Check sheet for the modelled part. Datum: model origin and axes. Units: mm. A direction names the side the tool comes from. Give positions to 0.01 mm unless a question says otherwise; leave off trailing zeros. Write each question's results on one line, items separated by ' | '. Start each with the question number.
1. Tool access check on faces 1 (the face through (88, 34, -49)), 2 (the face through (90, 26, -49)), 3 (the face through (52, 45.7, -49)). Record the directions out of +Z, -Z, +X, -X, +Y, -Y that give a thin tool (end or side, any length) a straight path to the whole face; none if there is none.
2. Material ranges on L1, parallel to Y at x = 77.5, z = -93.5; L2, parallel to Y at x = 47, z = -74.5; L3, parallel to Y at x = 59, z = -47.5, recorded low to high. Write a range as from..to.
3. Gauge pin test, flat ends, axial feed: pin 1 Ø6 at (x, y) = (82, 16) entering from -Z; pin 2 Ø10 at (x, z) = (56, -46.5) entering from +Y; pin 3 Ø2 at (y, z) = (3, -56) entering from -X; pin 4 Ø1.6 at (x, z) = (58.5, -64) entering from +Y. Record the tip position at first contact, or that the pin passes through.
4. Mould release check, pull along Y, two halves, no side actions. Record for faces 4 (the face through (52.82, 48, -49)), 5 (the face through (80, 1.83, -49)), 6 (the face through (87, 50.35, -49)): +Y half, -Y half, draft (parallel to the pull), parting line (faces both ways), or undercut.
from build123d import *

# Parameters (mm, degrees)
BOSS_EXTRUDE1_DEPTH = 100


with BuildPart() as part:
    # Sketch2 → Boss-Extrude1 (new body)
    with BuildSketch(Plane(origin=(0, 0, 0), x_dir=(-1, 0, 0), z_dir=(0, 0, -1))):
        with BuildLine():
            Line((-81.1, 43.92), (-46.615, 43.92))
            Line((-46.615, 43.92), (-46.615, 45.7))
            Line((-46.615, 45.7), (-49, 45.7))
            Line((-49, 45.7), (-49, 48.57))
            Line((-49, 48.57), (-45, 48.57))
            Line((-45, 48.57), (-45, 50.35))
            Line((-45, 50.35), (-50.82, 50.35))
            Line((-50.82, 50.35), (-50.82, 45.7))
            Line((-50.82, 45.7), (-52.82, 45.7))
            Line((-52.82, 45.7), (-52.82, 50.35))
            Line((-52.82, 50.35), (-54.224444444, 50.35))
            Line((-54.224444444, 50.35), (-54.224444444, 45.7))
            Line((-54.224444444, 45.7), (-56.224444444, 45.7))
            Line((-56.224444444, 45.7), (-56.224444444, 50.35))
            Line((-56.224444444, 50.35), (-57.628888889, 50.35))
            Line((-57.628888889, 50.35), (-57.628888889, 45.7))
            Line((-57.628888889, 45.7), (-59.628888889, 45.7))
            Line((-59.628888889, 45.7), (-59.628888889, 50.35))
            Line((-59.628888889, 50.35), (-61.033333333, 50.35))
            Line((-61.033333333, 50.35), (-61.033333333, 45.7))
            Line((-61.033333333, 45.7), (-63.033333333, 45.7))
            Line((-63.033333333, 45.7), (-63.033333333, 50.35))
            Line((-63.033333333, 50.35), (-64.437777778, 50.35))
            Line((-64.437777778, 50.35), (-64.437777778, 45.7))
            Line((-64.437777778, 45.7), (-66.437777778, 45.7))
            Line((-66.437777778, 45.7), (-66.437777778, 50.35))
            Line((-66.437777778, 50.35), (-67.842222222, 50.35))
            Line((-67.842222222, 50.35), (-67.842222222, 45.7))
            Line((-67.842222222, 45.7), (-69.842222222, 45.7))
            Line((-69.842222222, 45.7), (-69.842222222, 50.35))
            Line((-69.842222222, 50.35), (-71.246666667, 50.35))
            Line((-71.246666667, 50.35), (-71.246666667, 45.7))
            Line((-71.246666667, 45.7), (-73.246666667, 45.7))
            Line((-73.246666667, 45.7), (-73.246666667, 50.35))
            Line((-73.246666667, 50.35), (-74.651111111, 50.35))
            Line((-74.651111111, 50.35), (-74.651111111, 45.7))
            Line((-74.651111111, 45.7), (-76.651111111, 45.7))
            Line((-76.651111111, 45.7), (-76.651111111, 50.35))
            Line((-76.651111111, 50.35), (-78.055555556, 50.35))
            Line((-78.055555556, 50.35), (-78.055555556, 45.7))
            Line((-78.055555556, 45.7), (-80.055555556, 45.7))
            Line((-80.055555556, 45.7), (-80.055555556, 50.35))
            Line((-80.055555556, 50.35), (-81.46, 50.35))
            Line((-81.46, 50.35), (-81.46, 46.490680448))
            Line((-81.46, 46.490680448), (-83.46, 47.61664944))
            Line((-83.46, 47.61664944), (-83.46, 50.35))
            Line((-83.46, 50.35), (-90, 50.35))
            Line((-90, 50.35), (-90, 0))
            Line((-90, 0), (-72.9, 0))
            Line((-72.9, 0), (-72.9, 1.83))
            Line((-72.9, 1.83), (-74.3, 1.83))
            Line((-74.3, 1.83), (-74.3, 4.2))
            Line((-74.3, 4.2), (-67.3, 4.2))
            Line((-67.3, 4.2), (-67.3, 1.83))
            Line((-67.3, 1.83), (-68.7, 1.83))
            Line((-68.7, 1.83), (-68.7, 0))
            Line((-68.7, 0), (-45, 0))
            Line((-45, 0), (-45, 1.83))
            Line((-45, 1.83), (-65.3, 1.83))
            Line((-65.3, 1.83), (-65.3, 6.2))
            Line((-65.3, 6.2), (-77.73, 6.2))
            Line((-77.73, 6.2), (-77.73, 4.2))
            Line((-77.73, 4.2), (-76.3, 4.2))
            Line((-76.3, 4.2), (-76.3, 1.83))
            Line((-76.3, 1.83), (-83.3, 1.83))
            Line((-83.3, 1.83), (-83.3, 4.2))
            Line((-83.3, 4.2), (-81.87, 4.2))
            Line((-81.87, 4.2), (-81.87, 6.2))
            Line((-81.87, 6.2), (-84.76556902, 6.2))
            Line((-84.76556902, 6.2), (-85.557358859, 4.697239063))
            ThreePointArc((-85.557358859, 4.697239063), (-86.149971444, 2.200236409), (-86.836478439, 4.673072852))
            Line((-86.836478439, 4.673072852), (-88, 6.6925))
            Line((-88, 6.6925), (-86.26, 6.6925))
            Line((-86.26, 6.6925), (-86.26, 8.23))
            Line((-86.26, 8.23), (-88, 8.23))
            Line((-88, 8.23), (-88, 10.19))
            Line((-88, 10.19), (-86.26, 10.19))
            Line((-86.26, 10.19), (-86.26, 11.7275))
            Line((-86.26, 11.7275), (-88, 11.7275))
            Line((-88, 11.7275), (-88, 13.6875))
            Line((-88, 13.6875), (-86.26, 13.6875))
            Line((-86.26, 13.6875), (-86.26, 15.225))
            Line((-86.26, 15.225), (-88, 15.225))
            Line((-88, 15.225), (-88, 17.185))
            Line((-88, 17.185), (-86.26, 17.185))
            Line((-86.26, 17.185), (-86.26, 18.7225))
            Line((-86.26, 18.7225), (-88, 18.7225))
            Line((-88, 18.7225), (-88, 20.6825))
            Line((-88, 20.6825), (-86.26, 20.6825))
            Line((-86.26, 20.6825), (-86.26, 22.22))
            Line((-86.26, 22.22), (-88, 22.22))
            Line((-88, 22.22), (-88, 24.18))
            Line((-88, 24.18), (-86.26, 24.18))
            Line((-86.26, 24.18), (-86.26, 25.7175))
            Line((-86.26, 25.7175), (-88, 25.7175))
            Line((-88, 25.7175), (-88, 27.6775))
            Line((-88, 27.6775), (-86.26, 27.6775))
            Line((-86.26, 27.6775), (-86.26, 29.215))
            Line((-86.26, 29.215), (-88, 29.215))
            Line((-88, 29.215), (-88, 31.175))
            Line((-88, 31.175), (-86.26, 31.175))
            Line((-86.26, 31.175), (-86.26, 32.7125))
            Line((-86.26, 32.7125), (-88, 32.7125))
            Line((-88, 32.7125), (-88, 34.6725))
            Line((-88, 34.6725), (-86.26, 34.6725))
            Line((-86.26, 34.6725), (-86.26, 36.21))
            Line((-86.26, 36.21), (-88, 36.21))
            Line((-88, 36.21), (-88, 38.17))
            Line((-88, 38.17), (-86.26, 38.17))
            Line((-86.26, 38.17), (-86.26, 39.7075))
            Line((-86.26, 39.7075), (-88, 39.7075))
            Line((-88, 39.7075), (-88, 41.6675))
            Line((-88, 41.6675), (-86.26, 41.6675))
            Line((-86.26, 41.6675), (-86.26, 45.5))
            ThreePointArc((-86.26, 45.5), (-86.92871037, 47.968875623), (-85.105401522, 46.174978958))
            Line((-85.105401522, 46.174978958), (-81.1, 43.92))
        make_face()
    extrude(amount=BOSS_EXTRUDE1_DEPTH)


solid = part.part
Geometry says:
1) face 1: +Z, -Z, -X | face 2: +Z, -Z, +X, +Y, -Y | face 3: +Z, -Z, +Y
2) L1: 0..1.83, 4.2..6.2, 43.92..50.35 | L2: 0..1.83, 43.92..45.7, 48.57..50.35 | L3: 0..1.83, 43.92..45.7
3) pin 1: through | pin 2: y = 50.35 | pin 3: x = 65.3 | pin 4: y = 45.7
4) face 4: draft | face 5: undercut | face 6: +Y half
